Input: part model. Units: mm. Frame: model coordinates. A direction names the side the tool comes from. Coordinates: 2 decimals unless noted, no trailing zeros. Write each loop counter-clockwise with the first axis right and the second up, starting at its lowest first coordinate (ties: lowest second). Pieces come first, ordered by that corner, then holes. Notation, with made-up numbers: M 61.25,74 L 113.25,74 A5 cw 113.25,79 Z; hole C 17,62 d3. An arc over 180 degrees is marked long. Use one line per item in the form item = value.
from build123d import *

# Parameters (mm, degrees)
EXTRUDE_1_DEPTH = 5
EXTRUDE_2_DEPTH = 5


with BuildPart() as part:
    # 草图1 → 凸台-拉伸1 (new body)
    with BuildSketch(Plane(origin=(0, 0, 0), x_dir=(1, 0, 0), z_dir=(0, 1, 0))):
        with BuildLine():
            Line((-32, 0), (-30, 0))
            ThreePointArc((-30, 0), (0, 30), (30, 0))
            Line((30, 0), (32, 0))
            ThreePointArc((32, 0), (0, 32), (-32, 0))
        make_face()
    extrude(amount=EXTRUDE_1_DEPTH)

    # 草图2 → 凸台-拉伸2 (add)
    with BuildSketch(Plane(origin=(0, 0, 0), x_dir=(1, 0, 0), z_dir=(0, 1, 0))):
        Polygon((5, 52), (0, 52), (-5, 52), (-5, 31), (5, 31), align=None)
    extrude(amount=EXTRUDE_2_DEPTH)


solid = part.part
(1) Section query A-A on z = -22. Return the cut outline in (x, y).
Computed:
outline = M -23.24,0 L -20.4,0 L -20.4,5 L -23.24,5 Z; M 20.4,0 L 23.24,0 L 23.24,5 L 20.4,5 Z
(2) Section query B-B on y = 1.85. Return the cut outline in (x, z).
Computed:
outline = M -32,0 A32 ccw -5,-31.61 L -5,-52 L 5,-52 L 5,-31.61 A32 ccw 32,0 L 30,0 A30 cw -30,0 Z
(3) Set-up query: faces 4 (the flat face through (5, 2, -42)), 5 (the flat face through (0, 2, -52)), 6 (the flat face through (-5, 2, -42)). Return all of +Z, -Z, +X, -X, +Y, -Y with unobstructed straight access to the full face (end or side cutting, diameter ignored); none if empty.
Computed:
face_4 = -Z, +X, +Y, -Y
face_5 = -Z, +X, -X, +Y, -Y
face_6 = -Z, -X, +Y, -Y
(4) Section query C-C on z = -45.5. Return the cut outline in (x, y), plus the area to 3 significant figures.
Computed:
outline = M -5,0 L 5,0 L 5,5 L -5,5 Z
area = 50.0 mm^2
(5) Pull-direction query (X, two-part tool) for faces 1 (the flat face through (0, 0, -32)), 2 (the cylindrical face through (-0.66, 2.465, -29.993)), 3 (the cylindrical face through (-24.124, 2.465, -21.024)); classes: pulls with the +X half, pulls with the -X half, needs draft (parallel to the pull), parting line crosses it, or undercut.
Computed:
face_1 = needs draft
face_2 = undercut
face_3 = pulls with the -X half
(6) Line query: probe 1 along X at (y, z) = (2.3, -41); probe 2 along X at (y, z) = (2.9, -4.5); probe 3 along X at (y, z) = (3.7, -10.5). Output: solid intervals per line, ascending.
Computed:
probe_1 = -5 to 5
probe_2 = -31.68 to -29.66, 29.66 to 31.68
probe_3 = -30.23 to -28.1, 28.1 to 30.23
(7) First-contact query: pin 1 Ø1.5 at (y, z) = (1, -14) entering from +X; pin 2 Ø12 at (x, z) = (12.5, -30.5) entering from -Y; pin 3 Ø1.5 at (y, z) = (1, -43) entering from +X. Flat tips, straight axial feed; report the tip coordinate or a pass-through.
Computed:
pin_1 = 29.13
pin_2 = 0
pin_3 = 5
(8) Section query D-D on x = 0. Return the cut outline in (y, z), plus the area to 3 significant figures.
Computed:
outline = M 0,-52 L 5,-52 L 5,-30 L 0,-30 Z
area = 110 mm^2
